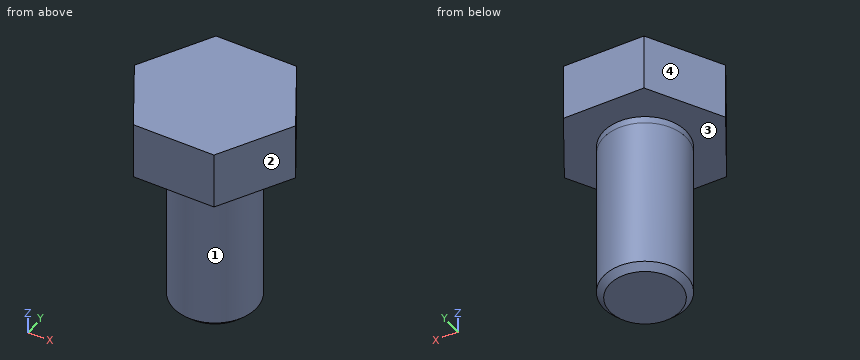
Solid Edge part; units mm, degrees
sketch "Sketch1" plane through (0, 0, 0) normal (0, 0, 1) x (1, 0, 0)
  circle A0 centre (0, 0) radius 5.8
extrude "Protrusion1" add sketch "Sketch1" along normal blind 4.15
sketch "Sketch2" plane through (0, 0, 0) normal (0, 0, -1) x (1, 0, 0)
  circle A0 centre (0, 0) radius 3
extrude "Protrusion2" add sketch "Sketch2" along normal blind 12
sketch "Sketch3" plane through (0, 0, -12) normal (0, 0, -1) x (1, 0, 0)
  circle A0 centre (0, 0) radius 2.9997
extrude "Cutout1" cut sketch "Sketch3" against normal blind 11.5 flip side to cut
chamfer "Chamfer_1" distance 0.45 angle 45 1 edges at (-2.9997, 0, -12)
sketch "Sketch4" plane through (0, 0, 4.15) normal (0, 0, 1) x (1, 0, 0)
  line L0 (-2.9394, 5) -> (2.9394, 5)
extrude "Cutout2" cut sketch "Sketch4" against normal up to next material side at (0, 5.05, 4.15)
pattern_circular "Pattern1" count 6 over 360 about axis through (0, 0, 4.15) along (0, 0, 1) of "Cutout2"
properties part number "118623"
Design review of the part built by this model. Coordinates are the model's own, in mm. Face numbers are marked on the shaded views. Coordinates: 2 decimals unless noted, no trailing zeros. Write each loop counter-clockwise with the first axis right and the second up, starting at its lowest first coordinate (ties: lowest second). Pieces come first, ordered by that corner, then holes. Notation, with made-up numbers: (15.5, -15.75) - (59.5, -15.75) arc R22 ccw to (59.5, 1.25) - close; hole circle Ø9 at (64, 11). An arc over 180 degrees is marked (long way). Use one line per item in the form item = value.
Q1. Consider section D-D (x = -3.5). Write out the cut boundary in (y, z), plus the area to 3 significant figures.
Taken from the geometry:
outline = (-3.94, 0) - (3.94, 0) - (3.94, 4.15) - (-3.94, 4.15) - close
area = 32.7 mm^2
Q2. Consider section C-C (y = 3.75). Write out the cut boundary in (x, z).
Taken from the geometry:
outline = (-3.61, 0) - (3.61, 0) - (3.61, 4.15) - (-3.61, 4.15) - close
Q3. Insertion check: pin 1 Ø1.5 at (x, z) = (-2, -6.5) entering from +Y; pin 2 Ø6 at (y, z) = (3, -4) entering from +X; pin 3 Ø6 at (y, z) = (-0.5, -4) entering from -X. Each pin has a flat end and moves straight along its axis. Give the tip position at first contact, or say it passes through.
Taken from the geometry:
pin_1 = 2.73
pin_2 = 3
pin_3 = -3
Q4. The part is to be moulded in two halves that separate along Y. For the marked faces 1, 2, 3 and 4, say which applies: +Y half, -Y half, draft (parallel to the pull), parting line (faces both ways), or undercut.
Taken from the geometry:
face_1 = parting line
face_2 = -Y half
face_3 = draft
face_4 = +Y half
Q5. For probe 1 along Z at (x, y) = (-5, -0.5); probe 2 along Y at (x, z) = (0.5, -10.5); probe 3 along Y at (x, z) = (2, -0.75), list the stretches that pass through material, from the lowest coordinate up.
Taken from the geometry:
probe_1 = 0 to 4.15
probe_2 = -2.96 to 2.96
probe_3 = -2.24 to 2.24
Q6. Consider section B-B (z = -11). Write out the cut boundary in (x, y).
Taken from the geometry:
outline = circle Ø6 at (0, 0)
